The listing builds one solid part. Answer for the finished solid, in the listing's coordinates (mm). Face numbers are marked on the shaded views. A direction names the side the tool comes from. Coordinates: 2 decimals unless noted, no trailing zeros. Write each loop counter-clockwise with the first axis right and the second up, starting at its lowest first coordinate (ties: lowest second). Pieces come first, ordered by that corner, then holes.
from build123d import *

# Parameters (mm, degrees)
POCKET_DEPTH      = 0.001
POCKET_DEPTH_BACK = 6.001
PAD_DEPTH         = 1


with BuildPart() as part:
    # AdditivePipe: sweep along a path in Sketch
    with BuildLine(Plane.XY) as additivepipe_path:
        ThreePointArc((240, 0), (221.731088, 91.844024), (169.705627, 169.705627))
    # Sketch001 → AdditivePipe (sweep)
    with BuildSketch(Plane(origin=(240, 0, 0), x_dir=(1, 0, 0), z_dir=(0, -1, 0))):
        Polygon((-8, 0), (8, 0), (8, 1), (1, 1), (1, 6), (-1, 6), (-1, 1), (-8, 1), align=None)
    sweep(path=additivepipe_path.line, is_frenet=True)

    # Sketch002 → Pocket (cut, two sides)
    with BuildSketch(Plane.XY) as pocket_sk:
        Polygon((235, 0), (234.5, 6), (238.5, 6), (238, 0), align=None)
        Polygon((242, 0), (241.5, 6), (245.5, 6), (245, 0), align=None)
    extrude(amount=-POCKET_DEPTH, mode=Mode.SUBTRACT)
    extrude(pocket_sk.sketch, amount=POCKET_DEPTH_BACK, mode=Mode.SUBTRACT)

    # Sketch003 → Pad (join)
    with BuildSketch(Plane.XY):
        Polygon((162.63456, 169.705627), (164.75588, 171.826948), (167.937861, 167.937861), (166.523647, 166.523647), align=None)
        Polygon((169.705627, 176.776695), (167.584307, 174.655375), (171.473394, 171.473394), (172.887608, 172.887608), align=None)
    extrude(amount=PAD_DEPTH)


solid = part.part
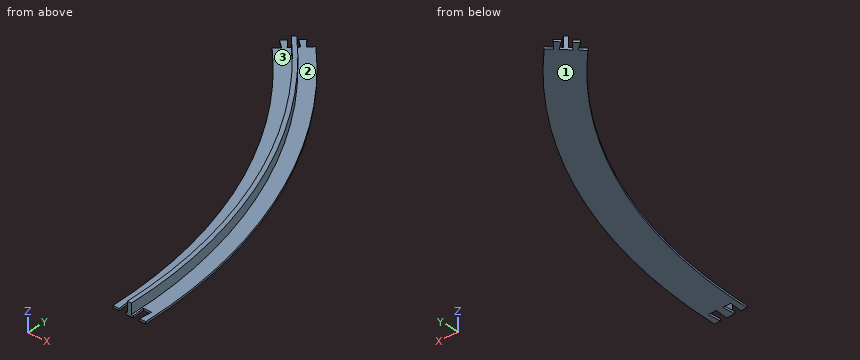
1. A tool of negligible diameter and unlimited length cuts with its end or side. For the marked faces 1, 2 and 3, from which of +Z, -Z, +X, -X, +Y, -Y can it reach the whole face along a straight path? Write none if from no direction.
Results found:
face 1: -Z, +X, -X, +Y, -Y
face 2: +Z, +X, +Y
face 3: +Z, -X, -Y
2. Flat-ended cylindrical pins translate along their axes: P1, Ø0.5, axis at x = 244.5, z = 0.5, coming from the -Y side; P2, Ø1.5, axis at y = 83, z = 3, coming from the -X side; P3, Ø3, axis at y = 22, z = 1, coming from the +X side. Find the tip coordinate at first contact, or state that the pin passes through.
Results found:
P1: stops at y = 6
P2: stops at x = 223.85
P3: stops at x = 247.15
3. Find the intervals of material crossed by L1, parallel to Z at x = 180.5, y = 151; L2, parallel to Y at x = 198.5, z = 5.55; L3, parallel to Y at x = 181.5, z = 0.6, in increasing order.
Results found:
L1: z = 0 to 1
L2: y = 133.11 to 136.67
L3: y = 144.51 to 169
4. Section C-C on z = 5.1 is taken. Give the vertices of the cut face in (x, y), then the cut area to 3 significant figures.
Results found:
outline: (169, 169) arc R239 cw to (239, 0) - (241, 0) arc R241 ccw to (170.41, 170.41) - close
area: 377 mm2
5. Section B-B on x = 194 is taken. Give the vertices of the cut face in (y, z), then the cut area to 3 significant figures.
Results found:
outline: (127.23, 0) - (154.49, 0) - (154.49, 1) - (142.99, 1) - (142.99, 6) - (139.59, 6) - (139.59, 1) - (127.23, 1) - close
area: 44.2 mm2
6. Section A-A on y = 25 is taken. Give the vertices of the cut face in (x, z), then the cut area to 3 significant figures.
Results found:
outline: (230.65, 0) - (246.74, 0) - (246.74, 1) - (239.7, 1) - (239.7, 6) - (237.69, 6) - (237.69, 1) - (230.65, 1) - close
area: 26.1 mm2
